Geometry check sheet. Reference: the model listing, model coordinates, mm. Face numbers are marked on the shaded views. A direction names the side the tool comes from. Coordinates: 2 decimals unless noted, no trailing zeros. Loops run counter-clockwise (first coordinate to the right, second up) from the corner with the lowest first, then second, coordinate; pieces in that order, holes last.
from build123d import *

# Parameters (mm, degrees)
F1_DEPTH = 70
F2_R     = 30.5
F3_DEPTH = 10
F5_DEPTH = 25


with BuildPart() as f1:
    # F0 (on Front) → F1 (new body)
    with BuildSketch(Plane.XZ):
        Polygon((1.617145, 13.06996), (-78.382855, 13.06996), (-78.382855, -11.93004), (-8.382855, 3.06996), (-8.382855, -11.93004), (1.617145, -11.93004), align=None)
    extrude(amount=F1_DEPTH)

    # F2 (on face) → F3 (cut)
    with BuildSketch(Plane.XY.offset(13.06996)):
        with Locations((-43.382855, -35)):
            Circle(F2_R)
    extrude(amount=-F3_DEPTH, mode=Mode.SUBTRACT)

    # F4 (on face) → F5 (cut)
    with BuildSketch(Plane.XY.offset(3.06996)):
        with BuildLine():
            ThreePointArc((-12.882855, -35), (-15.469745, -22.707389), (-22.791595, -12.5))
            Line((-22.791595, -12.5), (-63.974116, -12.5))
            ThreePointArc((-63.974116, -12.5), (-73.882855, -35), (-63.974116, -57.5))
            Line((-63.974116, -57.5), (-22.791595, -57.5))
            ThreePointArc((-22.791595, -57.5), (-15.469745, -47.292611), (-12.882855, -35))
        make_face()
    extrude(amount=-F5_DEPTH, mode=Mode.SUBTRACT)


solid = f1.part
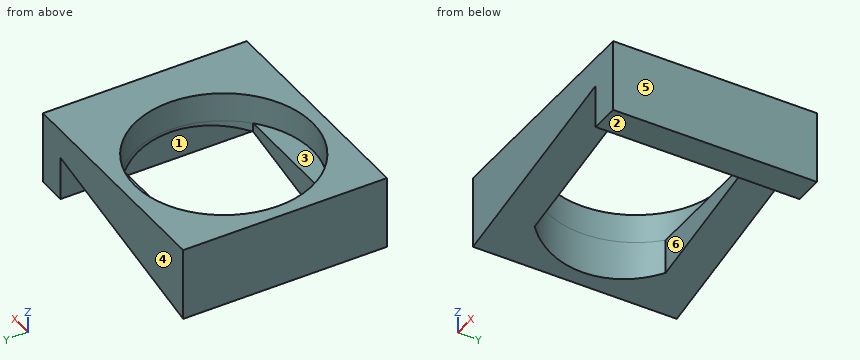
(1) Sectioned sample at C-C on y = -30.5. Record the cut outline in (x, z), and give its area (3 significant figures).
Findings:
outline: (-78.38, -11.93) - (-73.55, -10.89) - (-73.55, 13.07) - (-78.38, 13.07) - close; (-13.22, 2.03) - (-8.38, 3.07) - (-8.38, -11.93) - (1.62, -11.93) - (1.62, 13.07) - (-13.22, 13.07) - close
area: 419 mm2
(2) Sectioned sample at B-B on z = 10. Record the cut outline in (x, y).
Findings:
outline: (-78.38, -70) - (1.62, -70) - (1.62, 0) - (-78.38, 0) - close; hole circle Ø61 at (-43.38, -35)
(3) Scan lines: L1, parallel to Y at x = -23, z = 2; L2, parallel to X at y = -18.5, z = -5.75; L3, parallel to X at y = -24, z = 0.75. Record each from-to range of solid material in increasing order.
Findings:
L1: y = -70 to -57.5, -12.5 to 0
L2: x = -78.38 to -69.03, -8.38 to 1.62
L3: x = -78.38 to -71.83, -8.38 to 1.62
(4) Sectioned sample at A-A on x = -29. Record the cut outline in (y, z), and give its area (3 significant figures).
Findings:
outline: (-70, -1.35) - (-57.5, -1.35) - (-57.5, 3.07) - (-61.9, 3.07) - (-61.9, 13.07) - (-70, 13.07) - close; (-12.5, -1.35) - (0, -1.35) - (0, 13.07) - (-8.1, 13.07) - (-8.1, 3.07) - (-12.5, 3.07) - close
area: 273 mm2
(5) Access from +Z, -Z, +X, -X, +Y, -Y to the whole of each face (thin tool, end or side, straight path). Record for the marked faces 1, 2 and 3.
Findings:
face 1: -Z, +Y, -Y
face 2: -Z, +X, -X, +Y, -Y
face 3: +Z
(6) Draft check along X on the marked faces 4, 5 and 6. Enter one of: +X half, -X half, draft (parallel to the pull), parting line (faces both ways), or undercut.
Findings:
face 4: draft
face 5: +X half
face 6: undercut
(7) Sectioned sample at D-D on z = 1. Record the cut outline in (x, y).
Findings:
outline: (-78.38, -70) - (-18.04, -70) - (-18.04, -51.97) arc R30.5 cw to (-22.79, -57.5) - (-63.97, -57.5) arc R30.5 cw to (-63.97, -12.5) - (-22.79, -12.5) arc R30.5 cw to (-18.04, -18.03) - (-18.04, 0) - (-78.38, 0) - close; (-8.38, -70) - (1.62, -70) - (1.62, 0) - (-8.38, 0) - close
(8) Gauge pin test, flat end, axial feed: pin 1 Ø10 at (x, z) = (-36.5, 7.5) entering from +Y. Record the tip position at first contact, or that the pin passes through.
Findings:
pin 1: stops at y = 0
